from build123d import *

# Parameters (mm, degrees)
AUFSATZ_LINEAR_AUSTRAGEN1_DEPTH              = 22
AUFSATZ_LINEAR_AUSTRAGEN2_DEPTH              = 25
FORMSENKUNG_F_R_M4_LINSENSENKSCHRAUB_2_COUNT = 2
FORMSENKUNG_F_R_M4_LINSENSENKSCHRAUB_2_PITCH = 109
FORMSENKUNG_F_R_M4_LINSENSENKSCHRAUB_3_COUNT = 2
FORMSENKUNG_F_R_M4_LINSENSENKSCHRAUB_3_PITCH = 65
VERRUNDUNG1_R                                = 20
FASE1_SIZE                                   = 18


with BuildPart() as part:
    # Skizze1 → Aufsatz-Linear austragen1 (new body)
    with BuildSketch(Plane.XY):
        with BuildLine():
            Line((0, 0), (18, 0))
            Line((18, 0), (18, -142.266450527))
            ThreePointArc((18, -142.266450527), (24.940505875, -154.917322215), (39.339273926, -155.861067333))
            Line((39.339273926, -155.861067333), (115.937364916, -120.142790905))
            Line((115.937364916, -120.142790905), (126.502821459, -142.80048558))
            Line((126.502821459, -142.80048558), (3.113091309, -200.338061687))
            Line((3.113091309, -200.338061687), (1, -195.806522752))
            Line((1, -195.806522752), (1, -175))
            Line((1, -175), (1, -170))
            Line((1, -170), (0, -170))
            Line((0, -170), (0, 0))
        make_face()
    aufsatz_linear_austragen1 = extrude(amount=AUFSATZ_LINEAR_AUSTRAGEN1_DEPTH)

    # Skizze2 → Aufsatz-Linear austragen2 (add)
    with BuildSketch(Plane(origin=(77.289946844, -165.748825893, 0), x_dir=(0.9063077870366477, 0.4226182617407045, 0), z_dir=(0.4226182617407045, -0.9063077870366477, 0))):
        with BuildLine():
            Line((54.300399179, 22), (54.300399179, 65))
            Line((54.300399179, 65), (80.300399179, 65))
            Line((80.300399179, 65), (80.300399179, 26))
            ThreePointArc((80.300399179, 26), (72.68517549, 7.615223689), (54.300399179, 0))
            Line((54.300399179, 0), (54.300399179, 22))
        make_face()
    aufsatz_linear_austragen2 = extrude(amount=-AUFSATZ_LINEAR_AUSTRAGEN2_DEPTH)

    # Skizze6 → Formsenkung für M4 Linsensenkschraube mit Schlitz1 (revolve, cut)
    with BuildSketch(Plane(origin=(18, -32, 11), x_dir=(0, 0, -1), z_dir=(0, 1, 0))):
        Polygon((0, 0), (0, 18), (2.25, 18), (2.25, 2.45), (4.7, 0), align=None)
    formsenkung_f_r_m4_linsensenkschraube_mi = revolve(axis=Axis((24.35, -32, 11), (-1, 0, 0)), mode=Mode.SUBTRACT)

    # Formsenkung f_r M4 Linsensenkschraub 2: Formsenkung für M4 Linsensenkschraube mit Schlitz1 ×2
    with Locations(*[(0, -i * FORMSENKUNG_F_R_M4_LINSENSENKSCHRAUB_2_PITCH, 0) for i in range(1, FORMSENKUNG_F_R_M4_LINSENSENKSCHRAUB_2_COUNT)]):
        add(formsenkung_f_r_m4_linsensenkschraube_mi, mode=Mode.SUBTRACT)

    # Formsenkung f_r M4 Linsensenkschraub 3: Formsenkung für M4 Linsensenkschraube mit Schlitz1 ×2
    with Locations(*[(0, -i * FORMSENKUNG_F_R_M4_LINSENSENKSCHRAUB_3_PITCH, 0) for i in range(1, FORMSENKUNG_F_R_M4_LINSENSENKSCHRAUB_3_COUNT)]):
        add(formsenkung_f_r_m4_linsensenkschraube_mi, mode=Mode.SUBTRACT)

    # Spiegeln4: Aufsatz-Linear austragen2 across plane
    add(aufsatz_linear_austragen2.mirror(Plane(origin=(86.351068046, -56.694772515, 65), x_dir=(1, 0, 0), z_dir=(0, 0, -1))))

    # Spiegeln5: Aufsatz-Linear austragen1, Formsenkung für M4 Linsensenkschraube mit Schlitz1 across plane
    add(aufsatz_linear_austragen1.mirror(Plane.XY.offset(65)))
    add(formsenkung_f_r_m4_linsensenkschraube_mi.mirror(Plane.XY.offset(65)), mode=Mode.SUBTRACT)

    # Spiegeln5 copy 1 sketch → Spiegeln5 copy 1 (revolve, cut)
    with BuildSketch(Plane(origin=(18, -141, 119), x_dir=(0, 0, 1), z_dir=(0, 1, 0))):
        Polygon((0, 0), (0, -18), (2.25, -18), (2.25, -2.45), (4.7, 0), align=None)
    revolve(axis=Axis((24.35, -141, 119), (1, 0, 0)), mode=Mode.SUBTRACT)

    # Spiegeln5 copy 2 sketch → Spiegeln5 copy 2 (revolve, cut)
    with BuildSketch(Plane(origin=(18, -97, 119), x_dir=(0, 0, 1), z_dir=(0, 1, 0))):
        Polygon((0, 0), (0, -18), (2.25, -18), (2.25, -2.45), (4.7, 0), align=None)
    revolve(axis=Axis((24.35, -97, 119), (1, 0, 0)), mode=Mode.SUBTRACT)

    # Verrundung1
    verrundung1_edges = [part.edges().sort_by_distance(p)[0] for p in [
        (121.220093187, -131.471638242, 22),
        (121.220093187, -131.471638242, 108),
    ]]
    fillet(verrundung1_edges, radius=VERRUNDUNG1_R)

    # Fase1
    fase1_edges = [part.edges().sort_by_distance(p)[0] for p in [
        (18, 0, 119),
        (18, 0, 11),
    ]]
    chamfer(fase1_edges, length=FASE1_SIZE - 0.0001)  # a hair under: the kernel refuses the full size


solid = part.part
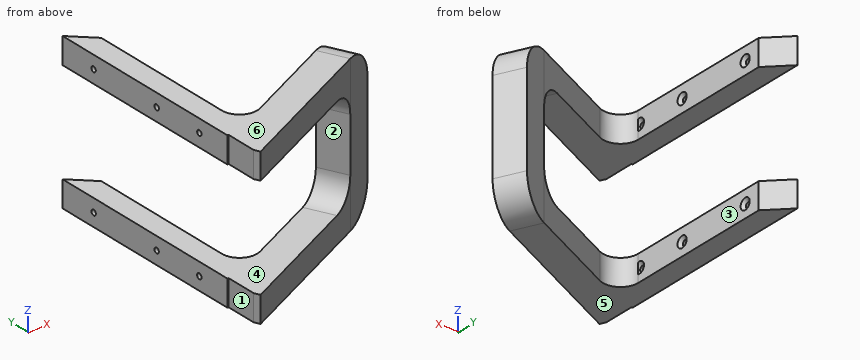
The model under review builds one solid part; all positions refer to its coordinate system, in mm. Face numbers are marked on the shaded views. A direction names the side the tool comes from. Give positions to 0.01 mm unless a question says otherwise; leave off trailing zeros. Write each loop counter-clockwise with the first axis right and the second up, starting at its lowest first coordinate (ties: lowest second). Pieces come first, ordered by that corner, then holes.
1. Add section B-B, the plane x = 92. Write out the cut boundary in (y, z).
2. Draft analysis for pull direction Z (two halves, no side actions). For the marked faces 4, 5 and 6, state which applies: +Z half, -Z half, draft (parallel to the pull), parting line (faces both ways), or undercut.
3. For P1, Ø4, axis at y = -141, z = 11, coming from the +X side; P2, Ø6.5, axis at y = -185, z = 118, coming from the -X side; P3, Ø0.5, axis at x = 0.5, z = 16, coming from the -Y side; P4, Ø2.5, axis at y = -32, z = 11, coming from the -X side, all flat-tipped, find the tip position at first contact; note any pin that passes through.
4. Wall thickness on L1, parallel to Z at x = 8, y = -97; L2, parallel to Y at x = 5.25, z = 119; L3, parallel to Y at x = 10.75, z = 119: over which ranges is each line inside the solid? List them lowest first.
5. Add section A-A, the plane y = -43. Write out the cut boundary in (x, z), plus the area to 3 significant figures.
6. Tool access review of the marked faces 1, 2 and 3: name each direction out of +Z, -Z, +X, -X, +Y, -Y from which nothing blocks a thin tool from reaching the whole face with its end or side.
Worked answers:
1. outline: (-158.89, 0) - (-131.3, 0) - (-131.3, 22) - (-158.89, 22) - close; (-158.89, 108) - (-131.3, 108) - (-131.3, 130) - (-158.89, 130) - close
2. face 4: undercut
2. face 5: -Z half
2. face 6: +Z half
3. P1: stops at x = 134.65
3. P2: stops at x = 1
3. P3: stops at y = -170
3. P4: passes through
4. L1: z = 0 to 8.75, 13.25 to 22, 108 to 116.75, 121.25 to 130
4. L2: y = -199.34 to -143.25, -138.75 to -99.25, -94.75 to -34.25, -29.75 to -5.25
4. L3: y = -196.78 to -143.25, -138.75 to -99.25, -94.75 to -34.25, -29.75 to -10.75
5. outline: (0, 0) - (18, 0) - (18, 22) - (0, 22) - close; (0, 108) - (18, 108) - (18, 130) - (0, 130) - close
5. area: 792 mm2
6. face 1: +Z, -Z, -X, -Y
6. face 2: -X, -Y
6. face 3: +Z, -Z, +Y
